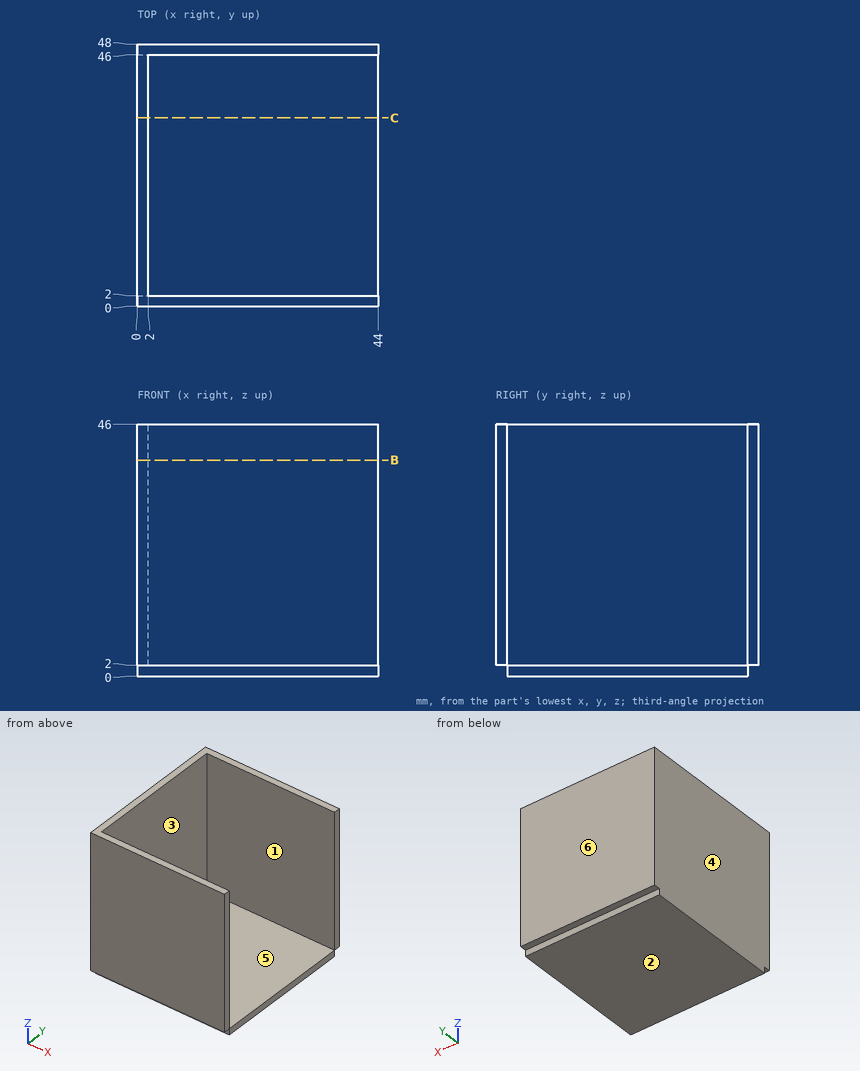
Can you work these out from the drawing? Everything is in mm from the part's minimum corner. A direction names the side the tool comes from. Round coordinates to 2 decimals unless told otherwise and drop trailing zeros. Write each loop counter-clockwise with the first axis right and the second up, starting at its lowest first coordinate (ties: lowest second). Pieces come first, ordered by that corner, then holes. Notation, with made-up numbers: M 53.5,-17 L 90.5,-17 A27 ccw 90.5,5 Z; hole C 49.25,-9.5 d6. An arc over 180 degrees is marked long. Use a Markdown table: item, result.
Item 1: Which directions (+Z, -Z, +X, -X, +Y, -Y) give clear straight access to the entire face, cutting with the end or side of a thin tool? Please do the marked faces 1 and 2.
Found:
| item | result |
|---|---|
| face 1 | +Z, +X |
| face 2 | -Z, +X, -X, +Y, -Y |
Item 2: We'd pull the mould along Y, two halves only. Please class the marked faces 3, 4, 5 and 6: released by +Y, released by -Y, zero draft, split by the parting line, or undercut.
Found:
| item | result |
|---|---|
| face 3 | undercut |
| face 4 | zero draft |
| face 5 | undercut |
| face 6 | released by +Y |
Item 3: If I drill on line 1 along Y through (x, z) = (35.5, 36); line 2 along X through (y, z) = (4, 21), over which ranges is the centre line in solid material (lowest first)? Write a range as [from, to].
Found:
| item | result |
|---|---|
| line 1 | y = [0, 2], [46, 48] |
| line 2 | x = [0, 2] |
Item 4: I want a section at B-B (z = 39.5). List the corners of the cut face in (x, y) for me, and give its area (3 significant figures).
Found:
| item | result |
|---|---|
| outline | M 0,0 L 44,0 L 44,2 L 2,2 L 2,46 L 44,46 L 44,48 L 0,48 Z |
| area | 264 mm2 |
Item 5: For pin 1 Ø2 at (x, y) = (22, 0.5) entering from -Z; pin 2 Ø1.6 at (x, z) = (24, 1) entering from +Y; pin 3 Ø8 at (x, y) = (30, 13.5) entering from +Z, each with a flat end and sliding along its axis, tell me the tip position at first contact or that it passes through.
Found:
| item | result |
|---|---|
| pin 1 | stops at z = 2 |
| pin 2 | stops at y = 46 |
| pin 3 | stops at z = 2 |
Item 6: I want a section at C-C (y = 34.5). List the corners of the cut face in (x, z) for me.
Found:
| item | result |
|---|---|
| outline | M 0,0 L 44,0 L 44,2 L 2,2 L 2,46 L 0,46 Z |
